from build123d import *

# Parameters (mm, degrees)
SKETCH1_W           = 203.047872021
SKETCH1_H           = 105.284081788
SKETCH1_R           = 8.89
BOSS_EXTRUDE1_DEPTH = 12.7
SKETCH2_R           = 14.2875
CUT_EXTRUDE1_DEPTH  = 7.9375


with BuildPart() as part:
    # Sketch1 → Boss-Extrude1 (new body)
    with BuildSketch(Plane(origin=(0, 0, 0), x_dir=(1, 0, 0), z_dir=(0, 1, 0))):
        with Locations((-40.397463616, -0.578483966)):
            Rectangle(SKETCH1_W, SKETCH1_H)
        with Locations(Location((-100, 0, 0), (0, 0, 270))):
            Circle(SKETCH1_R, mode=Mode.SUBTRACT)
        with Locations(Location((0, 0, 0), (0, 0, 270))):
            Circle(SKETCH1_R, mode=Mode.SUBTRACT)
    extrude(amount=BOSS_EXTRUDE1_DEPTH)

    # Sketch2 → Cut-Extrude1 (cut)
    with BuildSketch(Plane(origin=(0, 0, 0), x_dir=(1, 0, 0), z_dir=(0, 1, 0))):
        with Locations(Location((-100, 0, 0), (0, 0, 270))):
            Circle(SKETCH2_R)
        with Locations(Location((0, 0, 0), (0, 0, 270))):
            Circle(SKETCH2_R)
    extrude(amount=CUT_EXTRUDE1_DEPTH, mode=Mode.SUBTRACT)


solid = part.part
Read the model definition and answer for the solid it produces. Units are mm, in the model's axes. A direction names the side the tool comes from. Coordinates: 2 decimals unless noted, no trailing zeros. Loops run counter-clockwise (first coordinate to the right, second up) from the corner with the lowest first, then second, coordinate; pieces in that order, holes last.
Q1. The part is cut by section A-A on z = 0. Write down the section's boundary in (x, y).
Q2. The part is cut by section B-B on x = -100. Write down the section's boundary in (y, z), and give its area (3 significant figures).
Q3. Each of these flat-tipped pins is pushed along its axis until it touches: pin 1 Ø5 at (x, z) = (-36, -10) entering from -Y; pin 2 Ø8.5 at (x, z) = (2.5, -6.5) entering from -Y. Where does it stop, or does it pass through?
Q4. The mould has two halves that part along Z. Classify faces 1 (the face through (-141.921, 6, 1)), 2 (the face through (-42, 6, -52.064)), 3 (the face through (-92.504, 10.285, 4.779)): +Z half, -Z half, draft (parallel to the pull), parting line (faces both ways), or undercut.
Q5. Which of the six approach directions +Z, -Z, +X, -X, +Y, -Y give full straight-line access (tool end or side, diameter ignored) to faces 4 (the face through (-6, 7.938, -7)), 5 (the face through (-42, 12.7, 0))?
Q6. The part is cut by section C-C on y = 5.25. Write down the section's boundary in (x, z) (1 decimal), and give its area (3 significant figures).
Q7. Consider probe 1 along X at (y, z) = (10.15, 0); probe 2 along X at (y, z) = (5.75, 0); probe 3 along Z at (x, y) = (0, 9.25). Determine where each line is inside the solid, lowest interval first.
Results below:
1. outline: (-141.92, 0) - (-114.29, 0) - (-114.29, 7.94) - (-108.89, 7.94) - (-108.89, 12.7) - (-141.92, 12.7) - close; (-91.11, 7.94) - (-85.71, 7.94) - (-85.71, 0) - (-14.29, 0) - (-14.29, 7.94) - (-8.89, 7.94) - (-8.89, 12.7) - (-91.11, 12.7) - close; (8.89, 7.94) - (14.29, 7.94) - (14.29, 0) - (61.13, 0) - (61.13, 12.7) - (8.89, 12.7) - close
2. outline: (0, -52.06) - (12.7, -52.06) - (12.7, -8.89) - (7.94, -8.89) - (7.94, -14.29) - (0, -14.29) - close; (0, 14.29) - (7.94, 14.29) - (7.94, 8.89) - (12.7, 8.89) - (12.7, 53.22) - (0, 53.22) - close
2. area: 1,030 mm2
3. pin 1: stops at y = 0
3. pin 2: stops at y = 7.94
4. face 1: draft
4. face 2: -Z half
4. face 3: undercut
5. face 4: -Y
5. face 5: +Z, -Z, +X, -X, +Y
6. outline: (-141.9, -52.1) - (61.1, -52.1) - (61.1, 53.2) - (-141.9, 53.2) - close; hole circle Ø28.6 at (-100, 0); hole circle Ø28.6 at (0, 0)
6. area: 20,100 mm2
7. probe 1: x = -141.92 to -108.89, -91.11 to -8.89, 8.89 to 61.13
7. probe 2: x = -141.92 to -114.29, -85.71 to -14.29, 14.29 to 61.13
7. probe 3: z = -52.06 to -8.89, 8.89 to 53.22
